The model under review builds one solid part; all positions refer to its coordinate system, in mm. Face numbers are marked on the shaded views. Coordinates: 2 decimals unless noted, no trailing zeros. Order: outer loops, then holes, each group sorted by start corner. A loop starts at its lowest first (then second) coordinate and runs counter-clockwise, first axis right, second up. Notation, with made-up numbers: (-26, -4.75) -> (-5, -4.75) arc R19 cw to (-5, 27.25) -> close; hole circle Ø11 at (4.5, 66). An arc over 180 degrees is marked (long way). Use one line per item in the form item = value. Start each with the question number.
(1) Mouldability with a two-part tool opening along Y and no side actions: class the marked faces 1, 2, 3 and 4 as +Y half, -Y half, draft (parallel to the pull), parting line (faces both ways), or undercut.
(2) Take a section at A-A (x = 7). State the section outline as (y, z) points.
(3) Wall thickness on line 1 along Z through (x, y) = (-11.5, -0.5); line 2 along X through (y, z) = (-4, 2.5); line 3 along Z through (x, y) = (-5.75, -6): over which ranges is each line inside the solid? List them lowest first.
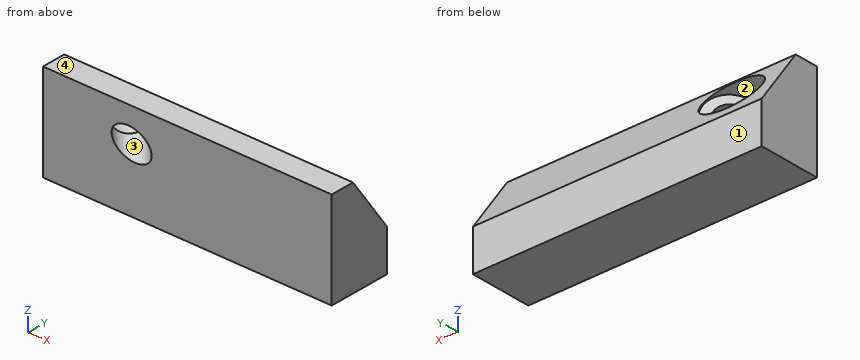
```python
from build123d import *

# Parameters (mm, degrees)
F0_W      = 30
F0_H      = 10
F1_DEPTH  = 6.5
F6_SIZE2  = 5.712592027
F6_SIZE   = 4
F9_R      = 1.5
F10_DEPTH = 12.5
F12_R     = 2.5
F13_DEPTH = 22


with BuildPart() as f1:
    # F0 (on Front) → F1 (new body)
    with BuildSketch(Plane.XZ):
        Rectangle(F0_W, F0_H)
    extrude(amount=F1_DEPTH)

    # F6
    f6_edges = [f1.edges().sort_by_distance(p)[0] for p in [
        (0, 0, 5),
    ]]
    f6_side = f1.faces().sort_by_distance((0, -3.25, 5))[0]
    chamfer(f6_edges, length=F6_SIZE, length2=F6_SIZE2, reference=f6_side)

    # F9 (on face) → F10 (cut, symmetric)
    with BuildSketch(Plane(origin=(0.2414814566, -0.25, -0.0647047613), x_dir=(-0.7304064958, -0.6612248329, -0.1711375799), z_dir=(-0.6830127019, 0.7071067812, 0.1830127019))):
        with Locations((8.2653104118, 3.1320350886)):
            Circle(F9_R)
    extrude(amount=F10_DEPTH, both=True, mode=Mode.SUBTRACT)

    # F12 (on face) → F13 (cut)
    with BuildSketch(Plane(origin=(-16.8338360907, 17.4276695297, 4.510612786), x_dir=(-0.7304064958, -0.6612248329, -0.1711375799), z_dir=(-0.6830127019, 0.7071067812, 0.1830127019))):
        with Locations((8.2653104118, 3.1320350886)):
            Circle(F12_R)
    extrude(amount=-F13_DEPTH, mode=Mode.SUBTRACT)


solid = f1.part
```
Findings:
q1.face_1 = +Y half
q1.face_2 = undercut
q1.face_3 = undercut
q1.face_4 = draft
q2.outline = (-6.5, -5) -> (0, -5) -> (0, -0.71) -> (-4, 5) -> (-6.5, 5) -> close
q3.line_1 = -5 to 0
q3.line_2 = -15 to -11.68, -6.27 to 15
q3.line_3 = -5 to 0.14, 3.09 to 5
